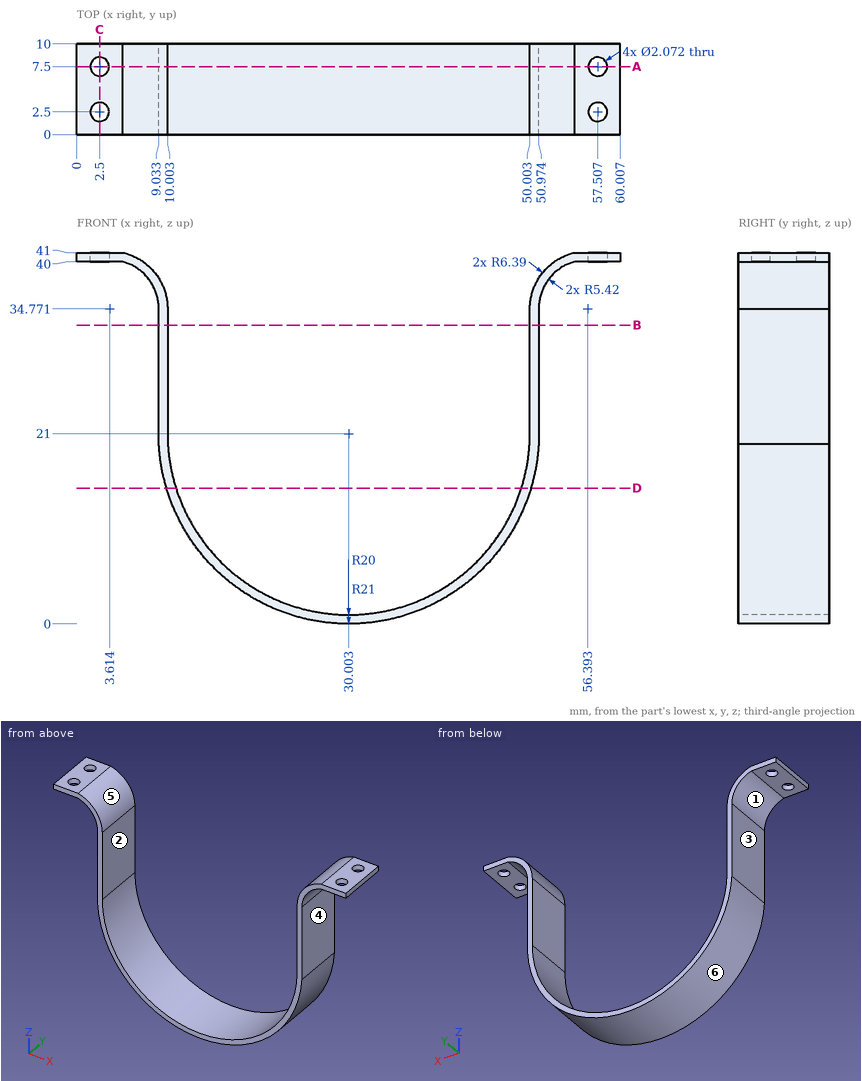
Answer from the drawing. Dimensions are ordinates in mm from the lowest x, y and z of the part. A direction names the side the tool comes from. Coordinates: 2 decimals unless noted, no trailing zeros. Loops run counter-clockwise (first coordinate to the right, second up) from the corner with the lowest first, then second, coordinate; pieces in that order, holes last.
Q1. The mould has two halves that part along X. Classify the marked faces 3, 4, 5 and 6: +X half, -X half, draft (parallel to the pull), parting line (faces both ways), or undercut.
Q2. The part is cut by section A-A on y = 7.5. Write down the section's boundary in (x, z), and give its area (3 significant figures).
Q3. The part is cut by section B-B on z = 33. Write down the section's boundary in (x, y), and give its area (3 significant figures).
Q4. Each of these flat-tipped pins is pushed along its axis until it touches: pin 1 Ø2 at (x, y) = (23.5, 5.5) entering from -Z; pin 2 Ø2.5 at (x, y) = (3, 3) entering from -Z; pin 3 Ø3 at (x, y) = (26, 2.5) entering from +Z; pin 4 Ø3.5 at (x, y) = (57.51, 7.5) entering from +Z. Where does it stop, or does it pass through?
Q5. Which of the six approach directions +Z, -Z, +X, -X, +Y, -Y give full straight-line access (tool end or side, diameter ignored) to the marked faces 1 and 2?
Q6. The part is cut by section C-C on x = 2.5. Write down the section's boundary in (y, z).
Q7. Consider probe 1 along Y at (x, z) = (2.5, 40.6); probe 2 along X at (y, z) = (4.75, 21.5); probe 3 along X at (y, z) = (8.5, 7.5) (1 decimal). Determine where each line is inside the solid, lowest interval first.
Q8. The part is cut by section D-D on z = 15. Write down the section's boundary in (x, y) (1 decimal).
Results below:
1. face 3: -X half
1. face 4: +X half
1. face 5: undercut
1. face 6: parting line
2. outline: (0, 40) - (1.46, 40) - (1.46, 41) - (0, 41) - close; (3.54, 40) - (5.04, 40) arc R5.42 cw to (9.03, 34.8) - (9.03, 19.88) arc R21 ccw to (50.97, 19.88) - (50.97, 34.8) arc R5.42 cw to (54.97, 40) - (56.47, 40) - (56.47, 41) - (54.97, 41) arc R6.39 ccw to (50, 34.8) - (50, 21) arc R20 cw to (10, 21) - (10, 34.8) arc R6.39 ccw to (5.04, 41) - (3.54, 41) - close; (58.54, 40) - (60.01, 40) - (60.01, 41) - (58.54, 41) - close
2. area: 112 mm2
3. outline: (9.03, 0) - (10, 0) - (10, 10) - (9.03, 10) - close; (50, 0) - (50.97, 0) - (50.97, 10) - (50, 10) - close
3. area: 19.4 mm2
4. pin 1: stops at z = 0.73
4. pin 2: stops at z = 40
4. pin 3: stops at z = 1.77
4. pin 4: stops at z = 41
5. face 1: -Z, -X, +Y, -Y
5. face 2: +Z, +Y, -Y
6. outline: (0, 40) - (1.46, 40) - (1.46, 41) - (0, 41) - close; (3.54, 40) - (6.46, 40) - (6.46, 41) - (3.54, 41) - close; (8.54, 40) - (10, 40) - (10, 41) - (8.54, 41) - close
7. probe 1: y = 0 to 1.46, 3.54 to 6.46, 8.54 to 10
7. probe 2: x = 9.03 to 10, 50 to 50.97
7. probe 3: x = 13.9 to 15.2, 44.8 to 46.1
8. outline: (9.9, 0) - (10.9, 0) - (10.9, 10) - (9.9, 10) - close; (49.1, 0) - (50.1, 0) - (50.1, 10) - (49.1, 10) - close
